Here's how the part is built. I have some questions about the finished solid (model axes, mm). Face numbers are marked on the shaded views. A direction names the side the tool comes from. Round coordinates to 2 decimals unless told otherwise and drop trailing zeros. Loops run counter-clockwise (first coordinate to the right, second up) from the corner with the lowest first, then second, coordinate; pieces in that order, holes last. Notation, with made-up numbers: (-32.5, -39) - (4.5, -39) arc R14 ccw to (4.5, -32) - close; hole circle Ø11 at (36, 87.25). An arc over 180 degrees is marked (long way). Return JSON: item names as keys, results as strings. Group by question number.
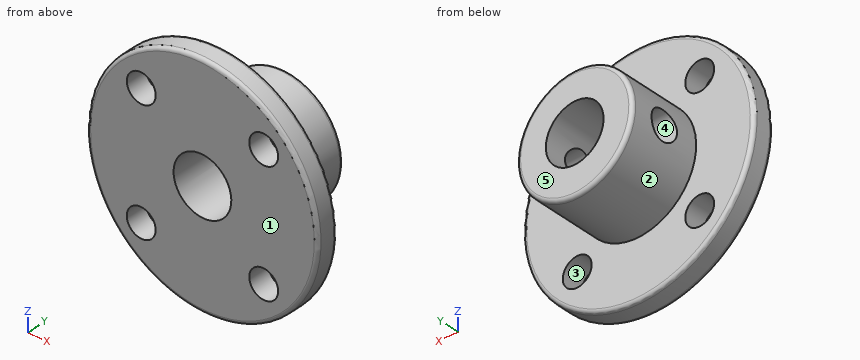
```python
from build123d import *

# Parameters (mm, degrees)
SKETCH1_R               = 16
BOSS_EXTRUDE1_DEPTH     = 3
SKETCH2_R               = 8
BOSS_EXTRUDE2_DEPTH     = 10
SKETCH3_R               = 4
CUT_EXTRUDE1_DEPTH      = 13
SKETCH4_R               = 2
CUT_EXTRUDE3_DEPTH      = 3
CUT_EXTRUDE4_DEPTH      = 10
CUT_EXTRUDE4_DEPTH_BACK = 24
SKETCH6_R               = 2
FILLET1_R               = 0.5
FILLET3_R               = 0.5


with BuildPart() as part:
    # Sketch1 → Boss-Extrude1 (new body)
    with BuildSketch(Plane(origin=(0, 0, 0), x_dir=(1, 0, 0), z_dir=(0, 1, 0))):
        with Locations(Location((0, 0, 0), (0, 0, 270))):
            Circle(SKETCH1_R)
    extrude(amount=BOSS_EXTRUDE1_DEPTH)

    # Sketch2 → Boss-Extrude2 (add)
    with BuildSketch(Plane(origin=(0, 3, 0), x_dir=(1, 0, 0), z_dir=(0, 1, 0))):
        with Locations(Location((0, 0, 0), (0, 0, 270))):
            Circle(SKETCH2_R)
    extrude(amount=BOSS_EXTRUDE2_DEPTH)

    # Sketch3 → Cut-Extrude1 (cut)
    with BuildSketch(Plane(origin=(0, 13, 0), x_dir=(1, 0, 0), z_dir=(0, 1, 0))):
        with Locations(Location((0, 0, 0), (0, 0, 270))):
            Circle(SKETCH3_R)
    extrude(amount=-CUT_EXTRUDE1_DEPTH, mode=Mode.SUBTRACT)

    # Sketch4 → Cut-Extrude3 (cut)
    with BuildSketch(Plane(origin=(0, 3, 0), x_dir=(1, 0, 0), z_dir=(0, 1, 0))):
        with Locations(Location((8.485281374, 8.485281374, 0), (0, 0, 270))):
            Circle(SKETCH4_R)
        with Locations(Location((8.485281374, -8.485281374, 0), (0, 0, 270))):
            Circle(SKETCH4_R)
        with Locations(Location((-8.485281374, -8.485281374, 0), (0, 0, 270))):
            Circle(SKETCH4_R)
        with Locations(Location((-8.485281374, 8.485281374, 0), (0, 0, 270))):
            Circle(SKETCH4_R)
    extrude(amount=-CUT_EXTRUDE3_DEPTH, mode=Mode.SUBTRACT)

    # Sketch6 → Cut-Extrude4 (cut, two sides: drawn at the far end of the back side and taken through both)
    with BuildSketch(Plane(origin=(0, 0, 0), x_dir=(0, 0, -1), z_dir=(1, 0, 0)).offset(-CUT_EXTRUDE4_DEPTH_BACK)):
        with Locations(Location((0, 8, 0), (0, 0, 180))):
            Circle(SKETCH6_R)
    extrude(amount=CUT_EXTRUDE4_DEPTH + CUT_EXTRUDE4_DEPTH_BACK, mode=Mode.SUBTRACT)

    # Fillet1
    fillet1_edges = [part.edges().sort_by_distance(p)[0] for p in [
        (0, 0, -16),
    ]]
    fillet(fillet1_edges, radius=FILLET1_R)

    # Fillet3
    fillet3_edges = [part.edges().sort_by_distance(p)[0] for p in [
        (0, 3, -16),
        (0, 13, -8),
    ]]
    fillet(fillet3_edges, radius=FILLET3_R)


solid = part.part
```
Q1. Will these pins go through, and if not, where does the flat tip stop? pin 1 Ø4.5 at (x, z) = (8.49, -8.49) entering from -Y; pin 2 Ø6 at (x, y) = (-2, 6.5) entering from -Z; pin 3 Ø4 at (x, y) = (-9.5, 4.5) entering from +Z; pin 4 Ø1.5 at (x, y) = (7.5, 3.5) entering from +Z.
Q2. Imagine slicing it at C-C, the plane y = 8. List the corners of the cut face in (x, z) for me.
Q3. For the marked faces 1 and 2, which set-ups out of +Z, -Z, +X, -X, +Y, -Y let a thin tool reach every point of the face, with its end or its side?
Q4. Please list where these lines run through material, in increasing order: line 1 (Y direction, x = 6.25, z = 0); line 2 (X direction, y = 4, z = 0); line 3 (X direction, y = 2, z = -7.5).
Q5. Imagine slicing it at B-B, the plane x = 0. List the corners of the cut face in (y, z) for me.
Q6. Imagine slicing it at D-D, the plane y = 11.25. List the corners of the cut face in (x, z) for me, and give its area (3 significant figures).
Q7. Imagine slicing it at A-A, the plane z = 0. List the corners of the cut face in (x, y) for me, and give its area (3 significant figures).
Q8. If we mould it in two halves opening along Y, with no side actions, what happens to the marked faces 3, 4 and 5? For each: +Y half, -Y half, draft (parallel to the pull), parting line (faces both ways), or undercut.
Output values:
{
 "1": {"pin 1": "stops at y = 0", "pin 2": "stops at z = -8", "pin 3": "stops at z = 13.47", "pin 4": "stops at z = 14.17"},
 "2": {"outline": "(-7.75, -2) arc R8 ccw to (7.75, -2) - (3.46, -2) arc R4 cw to (-3.46, -2) - close; (-7.75, 2) - (-3.46, 2) arc R4 cw to (3.46, 2) - (7.75, 2) arc R8 ccw to start"},
 "3": {"face 1": "+Z, -Z, +X, -X, -Y", "face 2": "+Y"},
 "4": {"line 1": "y = 0 to 6, 10 to 13", "line 2": "x = -8 to -4, 4 to 8", "line 3": "x = -14.13 to -10.23, -6.74 to 6.74, 10.23 to 14.13"},
 "5": {"outline": "(0, -15.5) arc R0.5 ccw to (0.5, -16) - (2.5, -16) arc R0.5 ccw to (3, -15.5) - (3, -8) - (12.5, -8) arc R0.5 ccw to (13, -7.5) - (13, -4) - (0, -4) - close; (0, 4) - (13, 4) - (13, 7.5) arc R0.5 ccw to (12.5, 8) - (3, 8) - (3, 15.5) arc R0.5 ccw to (2.5, 16) - (0.5, 16) arc R0.5 ccw to (0, 15.5) - close"},
 "6": {"outline": "circle Ø16 at (0, 0); hole circle Ø8 at (0, 0)", "area": "151 mm^2"},
 "7": {"outline": "(-16, 0.5) arc R0.5 ccw to (-15.5, 0) - (-4, 0) - (-4, 6) - (-8, 6) - (-8, 3) - (-15.5, 3) arc R0.5 ccw to (-16, 2.5) - close; (-8, 10) - (-4, 10) - (-4, 13) - (-7.5, 13) arc R0.5 ccw to (-8, 12.5) - close; (4, 0) - (15.5, 0) arc R0.5 ccw to (16, 0.5) - (16, 2.5) arc R0.5 ccw to (15.5, 3) - (8, 3) - (8, 6) - (4, 6) - close; (4, 10) - (8, 10) - (8, 12.5) arc R0.5 ccw to (7.5, 13) - (4, 13) - close", "area": "120 mm^2"},
 "8": {"face 3": "draft", "face 4": "undercut", "face 5": "+Y half"}
}
